For this review, take the finished solid that the model builds, in its own axes (mm). A direction names the side the tool comes from. Round coordinates to 2 decimals unless told otherwise and drop trailing zeros. Order: outer loops, then holes, each group sorted by start corner. A loop starts at its lowest first (then second) coordinate and runs counter-clockwise, first axis right, second up. Notation, with made-up numbers: (88.25, -29) - (133.25, -29) arc R32 cw to (133.25, 7) - close; hole circle Ø11 at (-20.75, 51.5). An arc over 180 degrees is marked (long way). One line per item, written item: value.
```python
from build123d import *

# Parameters (mm, degrees)
SKETCH1_R           = 2.5
BOSS_EXTRUDE1_DEPTH = 16
SKETCH2_R           = 4
BOSS_EXTRUDE2_DEPTH = 22
CHAMFER1_SIZE       = 0.5
FILLET1_R           = 0.5


with BuildPart() as part:
    # Sketch1 → Boss-Extrude1 (new body)
    with BuildSketch(Plane.XY):
        Circle(SKETCH1_R)
    extrude(amount=BOSS_EXTRUDE1_DEPTH)

    # Sketch2 → Boss-Extrude2 (add)
    with BuildSketch(Plane.XY.offset(16)):
        Circle(SKETCH2_R)
    extrude(amount=BOSS_EXTRUDE2_DEPTH)

    # Chamfer1
    chamfer1_edges = [part.edges().sort_by_distance(p)[0] for p in [
        (-2.5, 0, 0),
        (-4, 0, 16),
        (-4, 0, 38),
    ]]
    chamfer(chamfer1_edges, length=CHAMFER1_SIZE)

    # Fillet1
    fillet1_edges = [part.edges().sort_by_distance(p)[0] for p in [
        (-2.5, 0, 16),
    ]]
    fillet(fillet1_edges, radius=FILLET1_R)


solid = part.part
```
Item 1: Take a section at C-C (z = 26). Write out the cut boundary in (x, y), plus the area to 3 significant figures.
Returned:
outline: circle Ø8 at (0, 0)
area: 50.3 mm^2
Item 2: Machinability: for faces 1 (the flat face through (0, 0, 0)), 2 (the cylindrical face through (-0.54, -2.44, 7.9)), which of the approach directions +Z, -Z, +X, -X, +Y, -Y give a long, thin tool a straight path to every point of the face, cutting with its end or side? Answer none if there is none.
Returned:
face 1: -Z, +X, -X, +Y, -Y
face 2: -Z
Item 3: For P1, Ø1.5, axis at x = -2.5, z = 11.5, coming from the +Y side; P2, Ø4, axis at y = -3, z = 22.5, coming from the +X side; P3, Ø1.5, axis at y = -3, z = 17, coming from the -X side, all flat-tipped, find the tip position at first contact; note any pin that passes through.
Returned:
P1: y = 1.79
P2: x = 3.87
P3: x = -3.31
Item 4: Take a section at A-A (y = 0). Write out the cut boundary in (x, z).
Returned:
outline: (-4, 16.5) - (-3.5, 16) - (-3, 16) arc R0.5 cw to (-2.5, 15.5) - (-2.5, 0.5) - (-2, 0) - (2, 0) - (2.5, 0.5) - (2.5, 15.5) arc R0.5 cw to (3, 16) - (3.5, 16) - (4, 16.5) - (4, 37.5) - (3.5, 38) - (-3.5, 38) - (-4, 37.5) - close
Item 5: The part is to be moulded in two halves that separate along Y. For faces 3 (the cylindrical face through (-0.867, -3.905, 26.853)), 4 (the flat face through (3, 1, 16)), say which applies: +Y half, -Y half, draft (parallel to the pull), parting line (faces both ways), or undercut.
Returned:
face 3: parting line
face 4: draft
Item 6: Wall thickness on line 1 (Z direction, x = 2.5, y = -2); line 2 (Y direction, x = 0.25, z = 34.5); line 3 (X direction, y = -1.5, z = 33.5): over which ranges is each line inside the solid? List them lowest first.
Returned:
line 1: 16 to 38
line 2: -3.99 to 3.99
line 3: -3.71 to 3.71
